Design review of the part built by this model. Coordinates are the model's own, in mm. A direction names the side the tool comes from. Coordinates: 2 decimals unless noted, no trailing zeros. Use a Markdown table: item, result. Add a question column.
Q1. Draft analysis for pull direction Y (two halves, no side actions). For faces 1 (the face through (-2, -104.203, 52)), 2 (the face through (-137.5, 0, 93)), 3 (the face through (-2, 0, 105)), state which applies: pulls with the +Y half, pulls with the -Y half, needs draft (parallel to the pull), parting line crosses it, or undercut.
Q2. For faces 4 (the face through (-145, 20, 93)), 5 (the face through (-2, 100.797, 52)), list the 3-axis set-ups (+Z, -Z, +X, -X, +Y, -Y) from which the entire face can be reached by the end or side of a thin tool; tool diameter is ignored.
Q3. Clearance check with flat-ended pins moving along their axes: pin 1 Ø4.5 at (x, y) = (-141.5, 0.5) entering from +Z; pin 2 Ø4.5 at (y, z) = (-8, 89.5) entering from -X. State where each tip first meets the part, or that it passes through.
from build123d import *

# Parameters (mm, degrees)
F0_W     = 315
F0_H     = 205
F1_DEPTH = 105
F2_W     = 20
F2_H     = 40
F3_DEPTH = 20
F4_R     = 5


with BuildPart() as f1:
    # F0 (on Top) → F1 (new body)
    with BuildSketch(Plane.XY):
        with Locations((0, -1.702649286)):
            Rectangle(F0_W, F0_H)
    extrude(amount=F1_DEPTH)

    # F2 (on face) → F3 (cut)
    with BuildSketch(Plane.XY.offset(105)):
        with Locations((-147.5, 0)):
            Rectangle(F2_W, F2_H)
    extrude(amount=-F3_DEPTH, mode=Mode.SUBTRACT)

    # F4
    f4_edges = [f1.edges().sort_by_distance(p)[0] for p in [
        (0, -104.202649, 105),
        (157.5, -1.702649, 105),
        (0, 100.797351, 105),
        (-157.5, 60.398675, 105),
        (-157.5, -62.101325, 105),
        (-137.5, 0, 105),
        (-147.5, -20, 105),
        (-147.5, 20, 105),
        (157.5, -104.202649, 52.5),
        (157.5, 100.797351, 52.5),
        (157.5, -1.702649, 0),
        (0, -104.202649, 0),
        (-157.5, -104.202649, 52.5),
        (-157.5, 100.797351, 52.5),
        (0, 100.797351, 0),
        (-157.5, -1.702649, 0),
        (-157.5, 0, 85),
        (-157.5, 20, 95),
        (-157.5, -20, 95),
    ]]
    fillet(f4_edges, radius=F4_R)


solid = f1.part
Answer list:
| question | item | result |
|---|---|---|
| 1 | face 1 | pulls with the -Y half |
| 1 | face 2 | undercut |
| 1 | face 3 | needs draft |
| 2 | face 4 | +Z, -X |
| 2 | face 5 | +Z, -Z, +X, -X, +Y |
| 3 | pin 1 | z = 85 |
| 3 | pin 2 | x = -137.5 |
